```python
from build123d import *

# Parameters (mm, degrees)
SKETCH1_R           = 12.5
BOSS_EXTRUDE1_DEPTH = 17.6
SKETCH2_R           = 5.5
CUT_EXTRUDE1_DEPTH  = 50.8
SKETCH3_R           = 8
CUT_EXTRUDE3_DEPTH  = 15.6
CUT_EXTRUDE4_DEPTH  = 18.6
BOSS_EXTRUDE2_DEPTH = 17.6
FILLET1_R           = 2


with BuildPart() as part:
    # Sketch1 → Boss-Extrude1 (new body)
    with BuildSketch(Plane(origin=(0, 0, 0), x_dir=(1, 0, 0), z_dir=(0, 1, 0))):
        Circle(SKETCH1_R)
    extrude(amount=BOSS_EXTRUDE1_DEPTH)

    # Sketch2 → Cut-Extrude1 (cut)
    with BuildSketch(Plane(origin=(0, 17.6, 0), x_dir=(1, 0, 0), z_dir=(0, 1, 0))):
        Circle(SKETCH2_R)
    extrude(amount=-CUT_EXTRUDE1_DEPTH, mode=Mode.SUBTRACT)

    # Sketch3 → Cut-Extrude3 (cut)
    with BuildSketch(Plane(origin=(0, 17.6, 0), x_dir=(1, 0, 0), z_dir=(0, 1, 0))):
        Circle(SKETCH3_R)
    extrude(amount=-CUT_EXTRUDE3_DEPTH, mode=Mode.SUBTRACT)

    # Sketch4 → Cut-Extrude4 (cut, through all)
    with BuildSketch(Plane(origin=(0, 17.6, 0), x_dir=(1, 0, 0), z_dir=(0, 1, 0))):
        with BuildLine():
            ThreePointArc((-6.128355545, 5.142300877), (-0.697245942, 7.969557585), (5.142300877, 6.128355545))
            Line((5.142300877, 6.128355545), (8.034845121, 9.575555539))
            ThreePointArc((8.034845121, 9.575555539), (-1.089446784, 12.452433726), (-9.575555539, 8.034845121))
            Line((-9.575555539, 8.034845121), (-6.128355545, 5.142300877))
        make_face()
    extrude(amount=-CUT_EXTRUDE4_DEPTH, mode=Mode.SUBTRACT)

    # Sketch5 → Boss-Extrude2 (add, through all)
    with BuildSketch(Plane(origin=(0, 17.6, 0), x_dir=(1, 0, 0), z_dir=(0, 1, 0))):
        with BuildLine():
            Line((29.863521208, 8.997262141), (20.411315049, 20.106230978))
            Line((20.411315049, 20.106230978), (8.034845121, 9.575555539))
            ThreePointArc((8.034845121, 9.575555539), (12.499926406, 0.042893271), (8.100371818, -9.520187835))
            Line((8.100371818, -9.520187835), (29.863521208, 8.997262141))
        make_face()
    extrude(amount=-BOSS_EXTRUDE2_DEPTH)

    # Fillet1
    fillet1_edges = [part.edges().sort_by_distance(p)[0] for p in [
        (5.142300877, 9.8, -6.128355545),
        (-6.128355545, 9.8, -5.142300877),
    ]]
    fillet(fillet1_edges, radius=FILLET1_R)


solid = part.part
```
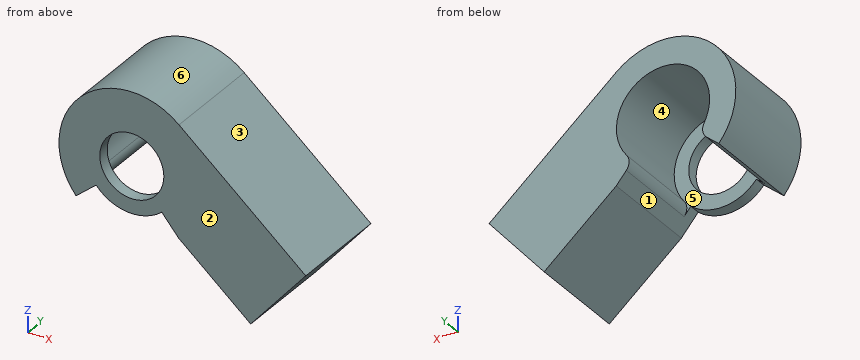
The model under review builds one solid part; all positions refer to its coordinate system, in mm. Face numbers are marked on the shaded views. A direction names the side the tool comes from. Round coordinates to 2 decimals unless told otherwise and drop trailing zeros. Order: outer loops, then holes, each group sorted by start corner. A loop starts at its lowest first (then second) coordinate and runs counter-clockwise, first axis right, second up. Notation, with made-up numbers: (36, 15.25) -> (91, 15.25) arc R28 cw to (91, 45.25) -> close; hole circle Ø7 at (-24, 86). An arc over 180 degrees is marked (long way). Use a Markdown table: item, result.
Q1. Tool access review of the marked faces 5 and 6: name each direction out of +Z, -Z, +X, -X, +Y, -Y from which nothing blocks a thin tool from reaching the whole face with its end or side.
Values:
| item | result |
|---|---|
| face 5 | +Y |
| face 6 | +Y, -Y |
Q2. We need section C-C on y = 1.5. Write out the cut boundary in (x, z), then the cut area to 3 significant figures.
Values:
| item | result |
|---|---|
| outline | (-9.58, -8.03) -> (-6.13, -5.14) arc R8 ccw to (5.14, -6.13) -> (8.03, -9.58) -> (20.41, -20.11) -> (29.86, -9) -> (8.1, 9.52) arc R12.5 ccw to start; hole circle Ø11 at (0, 0) |
| area | 592 mm^2 |
Q3. Mouldability with a two-part tool opening along Z and no side actions: class the marked faces 1, 2, 3 and 4 as +Z half, -Z half, draft (parallel to the pull), parting line (faces both ways), or undercut.
Values:
| item | result |
|---|---|
| face 1 | -Z half |
| face 2 | draft |
| face 3 | +Z half |
| face 4 | undercut |
Q4. For line 1 (Z direction, x = 0, y = 1); line 2 (X direction, y = 6.75, z = 0); line 3 (Y direction, x = -6, z = -3), list the stretches that pass through material, from the lowest coordinate up.
Values:
| item | result |
|---|---|
| line 1 | z = -8 to -5.5, 5.5 to 12.5 |
| line 2 | x = -12.5 to -8, 8 to 19.29 |
| line 3 | y = 0 to 2 |
Q5. We need section B-B on z = -1. Write out the cut boundary in (x, y).
Values:
| item | result |
|---|---|
| outline | (-12.46, 0) -> (-5.41, 0) -> (-5.41, 2) -> (-7.94, 2) -> (-7.94, 17.6) -> (-12.46, 17.6) -> close; (5.41, 0) -> (20.46, 0) -> (20.46, 17.6) -> (7.94, 17.6) -> (7.94, 2) -> (5.41, 2) -> close |
Q6. We need section D-D on y = 9.5. Write out the cut boundary in (x, z), then the cut area to 3 significant figures.
Values:
| item | result |
|---|---|
| outline | (-9.58, -8.03) -> (-7.51, -6.3) arc R2 ccw to (-7.03, -3.81) arc R8 cw (long way) to (6.26, -4.98) arc R2 ccw to (6.3, -7.51) -> (8.03, -9.58) -> (20.41, -20.11) -> (29.86, -9) -> (8.1, 9.52) arc R12.5 ccw to start |
| area | 484 mm^2 |
Q7. We need section A-A on x = 0. Write out the cut boundary in (y, z).
Values:
| item | result |
|---|---|
| outline | (0, -8) -> (2, -8) -> (2, -5.5) -> (0, -5.5) -> close; (0, 5.5) -> (2, 5.5) -> (2, 8) -> (17.6, 8) -> (17.6, 12.5) -> (0, 12.5) -> close |
Q8. Clearance check with flat-ended pins moving along their axes: P1, Ø10, axis at x = 0, z = 0, coming from the +Y side; P2, Ø4, axis at y = 10, z = -3, coming from the -X side; P3, Ø1, axis at y = 11, z = -8, coming from the +X side; P4, Ø4, axis at x = 5.5, y = 7, coming from the -Z side. State where each tip first meets the part, or that it passes through.
Values:
| item | result |
|---|---|
| P1 | passes through |
| P2 | stops at x = -12.46 |
| P3 | stops at x = 29.28 |
| P4 | stops at z = -8.94 |
